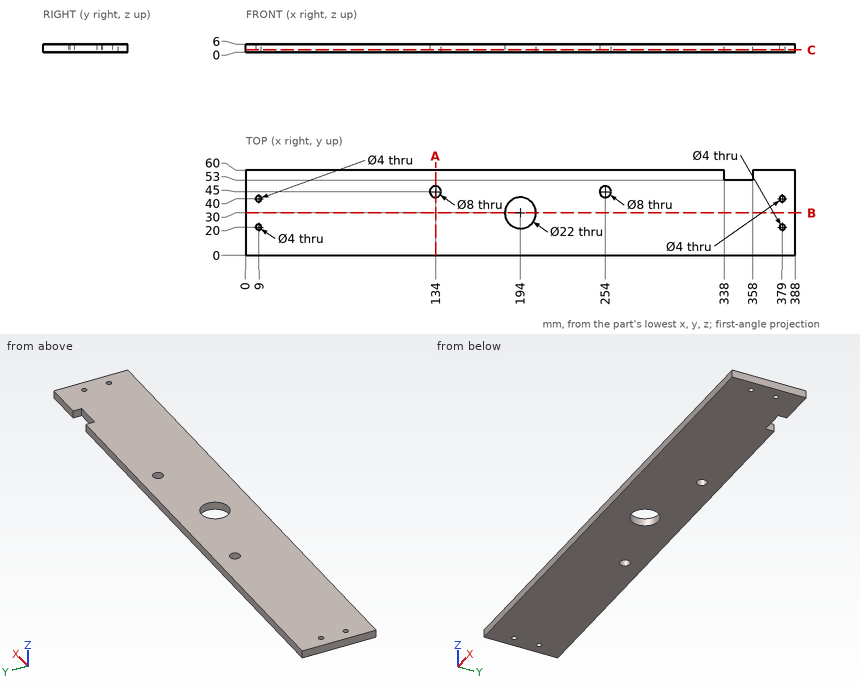
Study the drawing (mm; zero at the part's minimum x, y, z) and answer. Give positions to 0.01 mm unless a question says otherwise; leave off trailing zeros. Loops run counter-clockwise (first coordinate to the right, second up) from the corner with the lowest first, then second, coordinate; pieces in that order, holes last. Notation, with made-up numbers: (-30.5, -14.75) - (-9.5, -14.75) arc R18 ccw to (-9.5, 9.25) - close; hole circle Ø4 at (-15, -14). An arc over 180 degrees is marked (long way). Return JSON: item names as keys, results as strings. Group by question number.
1. Find section C-C (z = 1.85). Write down the section's boundary in (x, y), then the cut area to 3 significant figures.
2. Straight lines are drawn through the part: line 1 (Y direction, x = 379, z = 2.35); line 2 (Y direction, x = 194, z = 2.55); line 3 (X direction, y = 55.5, z = 2.9). For each, find the intervals that lie inside material, in ascending order. Write a range as [from, to].
3. Find section B-B (y = 30). Write down the section's boundary in (x, z).
4. Find section A-A (x = 134). Write down the section's boundary in (y, z).
Verdict:
{
 "1": {"outline": "(0, 0) - (388, 0) - (388, 60) - (358, 60) - (358, 53) - (338, 53) - (338, 60) - (0, 60) - close; hole circle Ø4 at (9, 20); hole circle Ø4 at (9, 40); hole circle Ø8 at (134, 45); hole circle Ø22 at (194, 30); hole circle Ø8 at (254, 45); hole circle Ø4 at (379, 20); hole circle Ø4 at (379, 40)", "area": "22,600 mm^2"},
 "2": {"line 1": "y = [0, 18], [22, 38], [42, 60]", "line 2": "y = [0, 19], [41, 60]", "line 3": "x = [0, 338], [358, 388]"},
 "3": {"outline": "(0, 0) - (183, 0) - (183, 6) - (0, 6) - close; (205, 0) - (388, 0) - (388, 6) - (205, 6) - close"},
 "4": {"outline": "(0, 0) - (41, 0) - (41, 6) - (0, 6) - close; (49, 0) - (60, 0) - (60, 6) - (49, 6) - close"}
}
